```python
from build123d import *

# Parameters (mm, degrees)
SKETCH1_W           = 47
SKETCH1_H           = 45.75
SKETCH1_R           = 1.6
BOSS_EXTRUDE1_DEPTH = 6
CUT_EXTRUDE1_DEPTH  = 7
FILLET1_R           = 5
SKETCH3_R           = 10.5
CUT_EXTRUDE2_DEPTH  = 7
SKETCH4_W           = 47
SKETCH4_H           = 6
BOSS_EXTRUDE2_DEPTH = 10
SKETCH6_R           = 1
CUT_EXTRUDE3_DEPTH  = 7


with BuildPart() as part:
    # Sketch1 → Boss-Extrude1 (new body)
    with BuildSketch(Plane(origin=(0, 0, 0), x_dir=(1, 0, 0), z_dir=(0, 1, 0))):
        with Locations((0, 22.875)):
            Rectangle(SKETCH1_W, SKETCH1_H)
        with Locations((-4.5, 41.25)):
            Circle(SKETCH1_R, mode=Mode.SUBTRACT)
        with Locations((-11.25, 21.25)):
            Circle(SKETCH1_R, mode=Mode.SUBTRACT)
        with Locations((11.25, 21.25)):
            Circle(SKETCH1_R, mode=Mode.SUBTRACT)
        with Locations((4.5, 41.25)):
            Circle(SKETCH1_R, mode=Mode.SUBTRACT)
    extrude(amount=BOSS_EXTRUDE1_DEPTH)

    # Sketch2 → Cut-Extrude1 (cut, through all)
    with BuildSketch(Plane(origin=(0, 6, 0), x_dir=(1, 0, 0), z_dir=(0, 1, 0))):
        Polygon((23.5, 32.53), (4.5, 45.75), (23.5, 45.75), align=None)
        Polygon((-23.5, 32.53), (-4.5, 45.75), (-23.5, 45.75), align=None)
    extrude(amount=-CUT_EXTRUDE1_DEPTH, mode=Mode.SUBTRACT)

    # Fillet1
    fillet1_edges = [part.edges().sort_by_distance(p)[0] for p in [
        (23.5, 3, -32.53),
        (4.5, 3, -45.75),
        (-23.5, 3, -32.53),
        (-4.5, 3, -45.75),
    ]]
    fillet(fillet1_edges, radius=FILLET1_R)

    # Sketch3 → Cut-Extrude2 (cut, through all)
    with BuildSketch(Plane.XZ):
        with Locations((11.25, -21.25)):
            Circle(SKETCH3_R)
    extrude(amount=-CUT_EXTRUDE2_DEPTH, mode=Mode.SUBTRACT)

    # Sketch4 → Boss-Extrude2 (add)
    with BuildSketch(Plane.XY):
        with Locations((0, 3)):
            Rectangle(SKETCH4_W, SKETCH4_H)
    extrude(amount=BOSS_EXTRUDE2_DEPTH)

    # Sketch6 → Cut-Extrude3 (cut, through all)
    with BuildSketch(Plane(origin=(0, 6, 0), x_dir=(1, 0, 0), z_dir=(0, 1, 0))):
        with Locations((-11.75, -5)):
            Circle(SKETCH6_R)
        with Locations((11.75, -5)):
            Circle(SKETCH6_R)
    extrude(amount=-CUT_EXTRUDE3_DEPTH, mode=Mode.SUBTRACT)


solid = part.part
```
Check sheet for the modelled part. Datum: model origin and axes. Units: mm. Round coordinates to 2 decimals unless told otherwise and drop trailing zeros. Loops run counter-clockwise (first coordinate to the right, second up) from the corner with the lowest first, then second, coordinate; pieces in that order, holes last. Notation, with made-up numbers: (50, 59) -> (56, 59) arc R22 ccw to (56, 70) -> close; hole circle Ø2 at (4, 43). An arc over 180 degrees is marked (long way). Answer in a Markdown table with one row per item.
Q1. Sectioned sample at C-C on z = -21.25. Enter the section's corners in (x, y).
Data:
| item | result |
|---|---|
| outline | (-23.5, 0) -> (-12.85, 0) -> (-12.85, 6) -> (-23.5, 6) -> close; (-9.65, 0) -> (0.75, 0) -> (0.75, 6) -> (-9.65, 6) -> close; (21.75, 0) -> (23.5, 0) -> (23.5, 6) -> (21.75, 6) -> close |
Q2. Release check for a two-part mould opening along Z. For faces 1 (the face through (23.5, 3, -10)), 2 (the face through (-12.43, 2.96, -22.33)), 3 (the face through (-22.95, 2.96, -32.2)) record: released by +Z, released by -Z, zero draft, split by the parting line, or undercut.
Data:
| item | result |
|---|---|
| face 1 | zero draft |
| face 2 | undercut |
| face 3 | released by -Z |
Q3. Sectioned sample at A-A on y = 2.6. Enter the section's corners in (x, z).
Data:
| item | result |
|---|---|
| outline | (-23.5, -29.92) arc R5 ccw to (-21.36, -34.02) -> (-5.79, -44.85) arc R5 ccw to (-2.93, -45.75) -> (2.93, -45.75) arc R5 ccw to (5.79, -44.85) -> (21.36, -34.02) arc R5 ccw to (23.5, -29.92) -> (23.5, 10) -> (-23.5, 10) -> close; hole circle Ø3.2 at (-11.25, -21.25); hole circle Ø2 at (-11.75, 5); hole circle Ø3.2 at (-4.5, -41.25); hole circle Ø21 at (11.25, -21.25); hole circle Ø3.2 at (4.5, -41.25); hole circle Ø2 at (11.75, 5) |
Q4. Sectioned sample at D-D on z = -15. Enter the section's corners in (x, y).
Data:
| item | result |
|---|---|
| outline | (-23.5, 0) -> (2.81, 0) -> (2.81, 6) -> (-23.5, 6) -> close; (19.69, 0) -> (23.5, 0) -> (23.5, 6) -> (19.69, 6) -> close |
Q5. Go/stop test with flat-tipped pins: P1, Ø24, axis at x = 11.25, z = -21.25, coming from the +Y side; P2, Ø3, axis at x = -7.5, y = 5, coming from the -Z side; P3, Ø1.9, axis at x = 4.5, z = -41.25, coming from the -Y side. Record where each tip stops, or that it passes through.
Data:
| item | result |
|---|---|
| P1 | stops at y = 6 |
| P2 | stops at z = -44.71 |
| P3 | passes through |
Q6. Thickness scan on L1, parallel to X at y = 2.8, z = 5; L2, parallel to Z at x = -11.75, y = 4.6; L3, parallel to Z at x = 11.75, y = 3.65. Record the ranges inside material, lowest first.
Data:
| item | result |
|---|---|
| L1 | x = -23.5 to -12.75, -10.75 to 10.75, 12.75 to 23.5 |
| L2 | z = -40.71 to -22.77, -19.73 to 4, 6 to 10 |
| L3 | z = -40.71 to -31.74, -10.76 to 4, 6 to 10 |
Q7. Sectioned sample at B-B on x = 19.5. Enter the section's corners in (y, z).
Data:
| item | result |
|---|---|
| outline | (0, -35.31) -> (6, -35.31) -> (6, -27.75) -> (0, -27.75) -> close; (0, -14.75) -> (6, -14.75) -> (6, 10) -> (0, 10) -> close |
